```python
from build123d import *

# Parameters (mm, degrees)
SKETCH1_W          = 1079.5
SKETCH1_H          = 63.5
EXTRUDE1_DEPTH     = 12.7
CUT_EXTRUDE1_DEPTH = 13.7
SKETCH6_R          = 2.0828
CUT_EXTRUDE3_DEPTH = 64.5
CUT_EXTRUDE4_DEPTH = 13.7000001
SKETCH8_R          = 2.0828
CUT_EXTRUDE5_DEPTH = 64.5


with BuildPart() as part:
    # Sketch1 → Extrude1 (new body)
    with BuildSketch(Plane.XY):
        with Locations((0, 996.95)):
            Rectangle(SKETCH1_W, SKETCH1_H)
    extrude(amount=EXTRUDE1_DEPTH)

    # Sketch4 → Cut-Extrude1 (cut, through all)
    with BuildSketch(Plane(origin=(0, 0, 0), x_dir=(-1, 0, 0), z_dir=(0, 0, -1))):
        with BuildLine():
            Line((-68.95, 1028.7), (-68.95, 995.9))
            ThreePointArc((-68.95, 995.9), (-63.95, 990.9), (-58.95, 995.9))
            Line((-58.95, 995.9), (-58.95, 1028.7))
            Line((-58.95, 1028.7), (-68.95, 1028.7))
        make_face()
        with BuildLine():
            Line((-351.05, 1028.7), (-361.05, 1028.7))
            Line((-361.05, 1028.7), (-361.05, 995.9))
            ThreePointArc((-361.05, 995.9), (-356.05, 990.9), (-351.05, 995.9))
            Line((-351.05, 995.9), (-351.05, 1028.7))
        make_face()
        with BuildLine():
            Line((58.95, 1028.7), (58.95, 995.9))
            ThreePointArc((58.95, 995.9), (63.95, 990.9), (68.95, 995.9))
            Line((68.95, 995.9), (68.95, 1028.7))
            Line((68.95, 1028.7), (58.95, 1028.7))
        make_face()
        with BuildLine():
            Line((351.05, 1028.7), (351.05, 995.9))
            ThreePointArc((351.05, 995.9), (356.05, 990.9), (361.05, 995.9))
            Line((361.05, 995.9), (361.05, 1028.7))
            Line((361.05, 1028.7), (351.05, 1028.7))
        make_face()
    extrude(amount=-CUT_EXTRUDE1_DEPTH, mode=Mode.SUBTRACT)

    # Sketch6 → Cut-Extrude3 (cut, through all)
    with BuildSketch(Plane.XZ.offset(-965.2)):
        with Locations((-356.05, 6.35)):
            Circle(SKETCH6_R)
        with Locations((356.05, 6.35)):
            Circle(SKETCH6_R)
        with Locations((63.95, 6.35)):
            Circle(SKETCH6_R)
        with Locations((-63.95, 6.35)):
            Circle(SKETCH6_R)
    extrude(amount=-CUT_EXTRUDE3_DEPTH, mode=Mode.SUBTRACT)

    # Sketch7 → Cut-Extrude4 (cut, through all)
    with BuildSketch(Plane.XY.offset(12.7)):
        with BuildLine():
            Line((-449.5, 995.9), (-449.5, 1028.7))
            Line((-449.5, 1028.7), (-439.5, 1028.7))
            Line((-439.5, 1028.7), (-439.5, 995.9))
            ThreePointArc((-439.5, 995.9), (-444.5, 990.9), (-449.5, 995.9))
        make_face()
        with BuildLine():
            Line((-500.3, 995.9), (-500.3, 1028.7))
            Line((-500.3, 1028.7), (-490.3, 1028.7))
            Line((-490.3, 1028.7), (-490.3, 995.9))
            ThreePointArc((-490.3, 995.9), (-495.3, 990.9), (-500.3, 995.9))
        make_face()
        with BuildLine():
            Line((490.3, 1028.7), (490.3, 995.9))
            ThreePointArc((490.3, 995.9), (495.3, 990.9), (500.3, 995.9))
            Line((500.3, 995.9), (500.3, 1028.7))
            Line((500.3, 1028.7), (490.3, 1028.7))
        make_face()
        with BuildLine():
            Line((439.5, 1028.7), (439.5, 995.9))
            ThreePointArc((439.5, 995.9), (444.5, 990.9), (449.5, 995.9))
            Line((449.5, 995.9), (449.5, 1028.7))
            Line((449.5, 1028.7), (439.5, 1028.7))
        make_face()
    extrude(amount=-CUT_EXTRUDE4_DEPTH, mode=Mode.SUBTRACT)

    # Sketch8 → Cut-Extrude5 (cut, through all)
    with BuildSketch(Plane.XZ.offset(-965.2)):
        with Locations((-495.3, 6.35)):
            Circle(SKETCH8_R)
        with Locations((-444.5, 6.35)):
            Circle(SKETCH8_R)
        with Locations((444.5, 6.35)):
            Circle(SKETCH8_R)
        with Locations((495.3, 6.35)):
            Circle(SKETCH8_R)
    extrude(amount=-CUT_EXTRUDE5_DEPTH, mode=Mode.SUBTRACT)


solid = part.part
```
Check sheet for the modelled part. Datum: model origin and axes. Units: mm. Coordinates: 2 decimals unless noted, no trailing zeros. Write item = value, one per line. Start each with the question number.
1. Go/stop test with a flat-tipped pin: pin 1 (3.5 mm diameter, centred on x = -444.5, z = 6.35, fed in from -Y) (3 decimals). Record where the tip stops, or that it passes through.
2. Sectioned sample at A-A (y = 1012). State how many separate pieces and enclosed holes the cut face has, then the cut area to 3 significant figures.
3. Thickness scan on probe 1 along Z at (x, y) = (495.3, 975.5); probe 2 along Y at (x, z) = (-496, 11.5); probe 3 along Z at (x, y) = (63, 975). Record the ranges inside material, lowest first.
The answers:
q1.pin_1 = through
q2.separate_pieces = 9
q2.enclosed_holes = 0
q2.area = 12,700 mm²
q3.probe_1 = 0 to 4.27, 8.43 to 12.7
q3.probe_2 = 965.2 to 990.95
q3.probe_3 = 0 to 4.5, 8.2 to 12.7
